Verification items for the finished model (mm, model axes). A direction names the side the tool comes from. Give positions to 0.01 mm unless a question says otherwise; leave off trailing zeros. Write each loop counter-clockwise with the first axis right and the second up, starting at its lowest first coordinate (ties: lowest second). Pieces come first, ordered by that corner, then holes. Notation, with made-up numbers: (-13, 24.5) -> (24, 24.5) arc R15 cw to (24, 30.5) -> close; hole circle Ø2 at (-35, 4.5). An arc over 180 degrees is marked (long way). Write item = value, one per line.
from build123d import *

# Parameters (mm, degrees)
SKETCH1_W                                    = 76.2
SKETCH1_H                                    = 38.1
BOSS_EXTRUDE1_DEPTH                          = 3.175
SKETCH4_R                                    = 1.5875
CUT_EXTRUDE1_DEPTH                           = 4.175
CBORE_FOR_2_PAN_HEAD_MACHINE_SCREW1_AT_COUNT = 2
CBORE_FOR_2_PAN_HEAD_MACHINE_SCREW1_AT_PITCH = 29.21
CBORE_FOR_2_PAN_HEAD_MACHINE_SCREW1_2_COUNT  = 2
CBORE_FOR_2_PAN_HEAD_MACHINE_SCREW1_2_PITCH  = 56.411450079
CBORE_FOR_2_PAN_HEAD_MACHINE_SCREW1_3_COUNT  = 2
CBORE_FOR_2_PAN_HEAD_MACHINE_SCREW1_3_PITCH  = 48.26
BOSS_EXTRUDE3_DEPTH                          = 1.27
FILLET1_R                                    = 6.35
FILLET2_R                                    = 0.635
FILLET3_R                                    = 0.635
F_6_CLEARANCE_HOLE1_D                        = 4.3053
CHAMFER1_SIZE                                = 0.508
CHAMFER2_SIZE                                = 0.254
CUT_EXTRUDE2_DEPTH                           = 2.27
SKETCH12_R                                   = 1.5875
BOSS_EXTRUDE4_DEPTH                          = 0.5


with BuildPart() as part:
    # Sketch1 → Boss-Extrude1 (new body)
    with BuildSketch(Plane.XY):
        Rectangle(SKETCH1_W, SKETCH1_H)
    extrude(amount=BOSS_EXTRUDE1_DEPTH)

    # Sketch4 → Cut-Extrude1 (cut, through all)
    with BuildSketch(Plane.XY.offset(3.175)):
        with Locations((24.13, -14.605)):
            Circle(SKETCH4_R)
        with Locations((24.13, 14.605)):
            Circle(SKETCH4_R)
        with Locations((-24.13, 14.605)):
            Circle(SKETCH4_R)
        with Locations((-24.13, -14.605)):
            Circle(SKETCH4_R)
    extrude(amount=-CUT_EXTRUDE1_DEPTH, mode=Mode.SUBTRACT)

    # Sketch7 → CBORE for #2 Pan Head Machine Screw1 (revolve, cut)
    with BuildSketch(Plane(origin=(24.13, 14.605, 0), x_dir=(0, 1, 0), z_dir=(1, 0, 0))):
        Polygon((0, 0), (0, 3.175), (1.35255, 3.175), (1.35255, 2.0828), (2.38125, 2.0828), (2.38125, 0.328717772), (2.667, 0), align=None)
    cbore_for_2_pan_head_machine_screw1 = revolve(axis=Axis((24.13, 14.605, -6.35), (0, 0, 1)), mode=Mode.SUBTRACT)

    # CBORE for #2 Pan Head Machine Screw1 at: CBORE for #2 Pan Head Machine Screw1 ×2
    with Locations(*[(0, -i * CBORE_FOR_2_PAN_HEAD_MACHINE_SCREW1_AT_PITCH, 0) for i in range(1, CBORE_FOR_2_PAN_HEAD_MACHINE_SCREW1_AT_COUNT)]):
        add(cbore_for_2_pan_head_machine_screw1, mode=Mode.SUBTRACT)

    # CBORE for _2 Pan Head Machine Screw1 2: CBORE for #2 Pan Head Machine Screw1 ×2
    with Locations(*[Vector(-0.855500079, -0.517802679, 0) * (i * CBORE_FOR_2_PAN_HEAD_MACHINE_SCREW1_2_PITCH) for i in range(1, CBORE_FOR_2_PAN_HEAD_MACHINE_SCREW1_2_COUNT)]):
        add(cbore_for_2_pan_head_machine_screw1, mode=Mode.SUBTRACT)

    # CBORE for _2 Pan Head Machine Screw1 3: CBORE for #2 Pan Head Machine Screw1 ×2
    with Locations(*[(-i * CBORE_FOR_2_PAN_HEAD_MACHINE_SCREW1_3_PITCH, 0, 0) for i in range(1, CBORE_FOR_2_PAN_HEAD_MACHINE_SCREW1_3_COUNT)]):
        add(cbore_for_2_pan_head_machine_screw1, mode=Mode.SUBTRACT)

    # Sketch5 → Boss-Extrude3 (add)
    with BuildSketch(Plane.XY.offset(3.175)):
        with BuildLine():
            ThreePointArc((-24.13, 11.176), (-21.705330847, 12.180330847), (-20.701, 14.605))
            Line((-20.701, 14.605), (-20.701, 17.526))
            Line((-20.701, 17.526), (20.701, 17.526))
            Line((20.701, 17.526), (20.701, 14.605))
            ThreePointArc((20.701, 14.605), (21.705330847, 12.180330847), (24.13, 11.176))
            Line((24.13, 11.176), (27.051, 11.176))
            Line((27.051, 11.176), (27.051, 9.461337048))
            ThreePointArc((27.051, 9.461337048), (26.858097964, 8.865714901), (26.35264224, 8.49626741))
            ThreePointArc((26.35264224, 8.49626741), (24.962639, 7.480286808), (24.4321584, 5.842325903))
            Line((24.4321584, 5.842325903), (24.4321584, -5.842325903))
            ThreePointArc((24.4321584, -5.842325903), (24.962639, -7.480286808), (26.35264224, -8.49626741))
            ThreePointArc((26.35264224, -8.49626741), (26.858097964, -8.865714901), (27.051, -9.461337048))
            Line((27.051, -9.461337048), (27.051, -11.176))
            Line((27.051, -11.176), (24.13, -11.176))
            ThreePointArc((24.13, -11.176), (21.705330847, -12.180330847), (20.701, -14.605))
            Line((20.701, -14.605), (20.701, -17.526))
            Line((20.701, -17.526), (-20.701, -17.526))
            Line((-20.701, -17.526), (-20.701, -14.605))
            ThreePointArc((-20.701, -14.605), (-21.705330847, -12.180330847), (-24.13, -11.176))
            Line((-24.13, -11.176), (-27.051, -11.176))
            Line((-27.051, -11.176), (-27.051, 11.176))
            Line((-27.051, 11.176), (-24.13, 11.176))
        make_face()
        with BuildLine():
            ThreePointArc((19.431, -14.605), (20.481131088, -11.644196619), (23.1621584, -10.006752112))
            Line((23.1621584, -10.006752112), (23.1621584, 10.006752112))
            ThreePointArc((23.1621584, 10.006752112), (20.481131088, 11.644196619), (19.431, 14.605))
            Line((19.431, 14.605), (19.431, 16.256))
            Line((19.431, 16.256), (-19.431, 16.256))
            Line((-19.431, 16.256), (-19.431, 14.605))
            ThreePointArc((-19.431, 14.605), (-20.807305235, 11.282305235), (-24.13, 9.906))
            Line((-24.13, 9.906), (-25.781, 9.906))
            Line((-25.781, 9.906), (-25.781, -9.906))
            Line((-25.781, -9.906), (-24.13, -9.906))
            ThreePointArc((-24.13, -9.906), (-20.807305235, -11.282305235), (-19.431, -14.605))
            Line((-19.431, -14.605), (-19.431, -16.256))
            Line((-19.431, -16.256), (19.431, -16.256))
            Line((19.431, -16.256), (19.431, -14.605))
        make_face(mode=Mode.SUBTRACT)
    extrude(amount=BOSS_EXTRUDE3_DEPTH)

    # Fillet1
    fillet1_edges = [part.edges().sort_by_distance(p)[0] for p in [
        (-38.1, 19.05, 1.5875),
        (38.1, 19.05, 1.5875),
        (38.1, -19.05, 1.5875),
        (-38.1, -19.05, 1.5875),
    ]]
    fillet(fillet1_edges, radius=FILLET1_R)

    # Fillet2
    fillet2_edges = [part.edges().sort_by_distance(p)[0] for p in [
        (-27.051, 11.176, 3.81),
        (-27.051, -11.176, 3.81),
        (-20.701, -17.526, 3.81),
        (20.701, -17.526, 3.81),
        (27.051, -11.176, 3.81),
        (27.051, 11.176, 3.81),
        (20.701, 17.526, 3.81),
        (-20.701, 17.526, 3.81),
    ]]
    fillet(fillet2_edges, radius=FILLET2_R)

    # Fillet3
    fillet3_edges = [part.edges().sort_by_distance(p)[0] for p in [
        (23.1621584, -10.006752112, 3.81),
        (19.431, -16.256, 3.81),
        (-19.431, -16.256, 3.81),
        (-25.781, -9.906, 3.81),
        (-25.781, 9.906, 3.81),
        (-19.431, 16.256, 3.81),
        (19.431, 16.256, 3.81),
        (23.1621584, 10.006752112, 3.81),
    ]]
    fillet(fillet3_edges, radius=FILLET3_R)

    # #6 Clearance Hole1 (through all)
    with Locations(Plane.XY.offset(3.175)):
        with Locations((-33.3375, 12.7), (-33.714363812, -11.954179128), (32.991908684, 14.039088205), (33.3375, -12.7)):
            Hole(F_6_CLEARANCE_HOLE1_D / 2)

    # Chamfer1
    chamfer1_edges = [part.edges().sort_by_distance(p)[0] for p in [
        (38.1, 0, 0),
        (-38.1, 0, 0),
        (0, 19.05, 0),
        (0, -19.05, 0),
        (-36.240128061, -17.190128061, 0),
        (-36.240128061, 17.190128061, 0),
        (36.240128061, 17.190128061, 0),
        (36.240128061, -17.190128061, 0),
    ]]
    chamfer(chamfer1_edges, length=CHAMFER1_SIZE)

    # Chamfer2
    chamfer2_edges = [part.edges().sort_by_distance(p)[0] for p in [
        (35.49015, -12.7, 3.175),
        (35.49015, -12.7, 0),
        (35.144558684, 14.039088205, 3.175),
        (35.144558684, 14.039088205, 0),
        (-31.561713812, -11.954179128, 3.175),
        (-31.561713812, -11.954179128, 0),
        (-31.18485, 12.7, 3.175),
        (-31.18485, 12.7, 0),
    ]]
    chamfer(chamfer2_edges, length=CHAMFER2_SIZE)

    # Sketch11 → Cut-Extrude2 (cut, through all)
    with BuildSketch(Plane.XY.offset(3.175)):
        with BuildLine():
            Line((24.4321584, 4.7625), (24.4321584, -4.7625))
            ThreePointArc((24.4321584, -4.7625), (23.7971584, -4.1275), (23.1621584, -4.7625))
            Line((23.1621584, -4.7625), (23.1621584, 4.7625))
            ThreePointArc((23.1621584, 4.7625), (23.7971584, 4.1275), (24.4321584, 4.7625))
        make_face()
    extrude(amount=CUT_EXTRUDE2_DEPTH, mode=Mode.SUBTRACT)

    # Sketch12 → Boss-Extrude4 (add)
    with BuildSketch(Plane(origin=(0, 0, 2.0828), x_dir=(-1, 0, 0), z_dir=(0, 0, -1))):
        with Locations((-24.13, 14.605)):
            Circle(SKETCH12_R)
        with Locations((24.13, 14.605)):
            Circle(SKETCH12_R)
        with Locations((24.13, -14.605)):
            Circle(SKETCH12_R)
        with Locations((-24.13, -14.605)):
            Circle(SKETCH12_R)
    extrude(amount=-BOSS_EXTRUDE4_DEPTH)


solid = part.part
Item 1: Sectioned sample at B-B on x = 1. Record the cut outline in (y, z) (3 decimals), then the cut area to 3 significant figures.
Response values:
outline = (-19.05, 0.508) -> (-18.542, 0) -> (18.542, 0) -> (19.05, 0.508) -> (19.05, 3.175) -> (17.526, 3.175) -> (17.526, 4.445) -> (16.256, 4.445) -> (16.256, 3.175) -> (-16.256, 3.175) -> (-16.256, 4.445) -> (-17.526, 4.445) -> (-17.526, 3.175) -> (-19.05, 3.175) -> close
area = 124 mm^2
Item 2: Sectioned sample at C-C on z = 1.2. Give the number of separate pieces and of enclosed holes in the cut face, then the cut area to 3 significant figures.
Response values:
separate_pieces = 1
enclosed_holes = 8
area = 2,740 mm^2
Item 3: Set-up check for faces 1 (the cylindrical face through (-36.29, 17.14, 1.86)), 2 (the cylindrical face through (21.679, 12.207, 3.801)), 3 (the cylindrical face through (20.37, 11.79, 3.8)): record each of +Z, -Z, +X, -X, +Y, -Y from which the full face is reachable in a straight line by a thin tool's end or side.
Response values:
face_1 = +Z, -Z, -X, +Y
face_2 = +Z, +X, +Y
face_3 = +Z
Item 4: Mould release check, pull along X, two halves, no side actions. Record for faces 4 (the cylindrical face through (-36.29, -17.14, 1.86)), 5 (the cylindrical face through (-31.63, 11.39, 1.57)), 6 (the flat face through (38.1, 0, 2)): +X half, -X half, draft (parallel to the pull), parting line (faces both ways), or undercut.
Response values:
face_4 = -X half
face_5 = undercut
face_6 = +X half
Item 5: Go/stop test with flat-tipped pins: P1, Ø1.4, axis at y = -8, z = 4, coming from the -X side; P2, Ø19, axis at x = 6, y = 2.5, coming from the +Z side (3 decimals); P3, Ø0.5, axis at y = 10, z = 4, coming from the +X side; P4, Ø4, axis at x = 32.99, y = 14.04, coming from the -Z side. Record where each tip stops, or that it passes through.
Response values:
P1 = -27.05
P2 = 3.175
P3 = 27.05
P4 = through
Item 6: Sectioned sample at A-A on y = 2.5. Record the cut outline in (x, z) (3 decimals), then the cut area to 3 significant figures.
Response values:
outline = (-38.1, 0.508) -> (-37.592, 0) -> (37.592, 0) -> (38.1, 0.508) -> (38.1, 3.175) -> (-25.781, 3.175) -> (-25.781, 4.445) -> (-27.051, 4.445) -> (-27.051, 3.175) -> (-38.1, 3.175) -> close
area = 243 mm^2
Item 7: Material ranges on line 1 (Y direction, x = 24.13, z = 2.7); line 2 (Y direction, x = 24.13, z = 0.9); line 3 (Y direction, x = 17, z = 3.6), recorded low to high.
Response values:
line_1 = -19.05 to -16.19, -13.02 to 13.02, 16.19 to 19.05
line_2 = -19.05 to -16.99, -12.22 to 12.22, 16.99 to 19.05
line_3 = -17.53 to -16.26, 16.26 to 17.53
Item 8: Sectioned sample at D-D on x = 28. Record the cut outline in (y, z) (3 decimals).
Response values:
outline = (-19.05, 0.508) -> (-18.542, 0) -> (18.542, 0) -> (19.05, 0.508) -> (19.05, 3.175) -> (-19.05, 3.175) -> close
